Autodesk Fusion 360 part; units mm, degrees
sketch "Sketch1" plane through (0, 0, 0) normal (0, 0, 1) x (1, 0, 0)
  line L0 (-25, 25) -> (25, 25)
  line L1 (25, 25) -> (25, -25)
  line L2 (25, -25) -> (-25, -25)
  line L3 (-25, -25) -> (-25, 25)
extrude "Extrude1" add sketch "Sketch1" along normal blind 5
sketch "Sketch2" plane through (0, 0, 5) normal (0, 0, 1) x (-1, 0, 0)
  line L0 (25, 25) -> (-25, 25)
  line L1 (-25, 25) -> (-25, -25)
  line L2 (-25, -25) -> (25, -25)
  line L3 (25, -25) -> (25, 25)
  circle A0 centre (0, 0) radius 4.5
  line L4 (0.0733, -4.4994) -> (0.0733, 4.4994)
  line L5 (4.5, 0) -> (-4.5, 0)
  dimension "d3" = 9
hole "Hole1" at (-4.5, 0, 5) direction (0, 0, -1) diameter 2.1 depth 11 tip angle 118 counterbore diameter 5 counterbore depth 2
pattern_circular "C-Pattern1" count 4 over 360 about axis through (0, 0, 1.75) along (0, 0, 1) of "Hole1"
extrude "Extrude2" add 1 faces at (-18.5157, 0.0262, 0) along direction (0, 0, -1) blind 2
extrude "Extrude3" cut 1 faces at (-18.5157, 0.0262, -2) along direction (0, 0, 1) blind 2
Geometry: final body of the model. Coordinates: model frame, mm. A direction names the side the tool comes from. Round coordinates to 2 decimals unless told otherwise and drop trailing zeros. Loops run counter-clockwise (first coordinate to the right, second up) from the corner with the lowest first, then second, coordinate; pieces in that order, holes last.
Item 1: Reachability of faces 1 (the flat face through (-3, 0, 3)), 2 (the cylindrical face through (3.46, -0.14, 1.52)) from +Z, -Z, +X, -X, +Y, -Y: full face, straight path, thin tool, end or side. Return the list, or none.
Checked values:
face 1: +Z
face 2: +Z, -Z
Item 2: Section B-B, the plane x = -4.5. Output: boundary loops of the cut face in (y, z).
Checked values:
outline: (-25, 0) - (-1.05, 0) - (-1.05, 3) - (-2.5, 3) - (-2.5, 5) - (-25, 5) - close; (1.05, 0) - (25, 0) - (25, 5) - (2.5, 5) - (2.5, 3) - (1.05, 3) - close
Item 3: Contact query for flat-ended pins moving along their axis: P1, Ø1.5, axis at x = -1, y = 4.5, coming from the +Z side; P2, Ø1.7, axis at x = 4.5, y = 0, coming from the +Z side. Output: stop coordinate, or through.
Checked values:
P1: stops at z = 3
P2: passes through
Item 4: Section A-A, the plane z = 4.2. Output: boundary loops of the cut face in (x, y).
Checked values:
outline: (-25, -25) - (25, -25) - (25, 25) - (-25, 25) - close; hole circle Ø5 at (-4.5, 0); hole circle Ø5 at (0, -4.5); hole circle Ø5 at (0, 4.5); hole circle Ø5 at (4.5, 0)
Item 5: Line query: L1, parallel to Y at x = 0, z = 1.3; L2, parallel to Y at x = 0, z = 4.45; L3, parallel to X at y = -4.5, z = 2.25. Output: solid intervals per line, ascending.
Checked values:
L1: y = -25 to -5.55, -3.45 to 3.45, 5.55 to 25
L2: y = -25 to -7, -2 to 2, 7 to 25
L3: x = -25 to -1.05, 1.05 to 25
Item 6: Mould query, pull axis X, two halves, no side actions, for faces 3 (the cylindrical face through (0, -7, 4)), 4 (the flat face through (25, 0, 3)), 5 (the flat face through (-25, 0, 3)), 6 (the cylindrical face through (-3.46, 0.14, 1.52)). Classes: released by +X, released by -X, zero draft, split by the parting line, or undercut.
Checked values:
face 3: undercut
face 4: released by +X
face 5: released by -X
face 6: undercut
